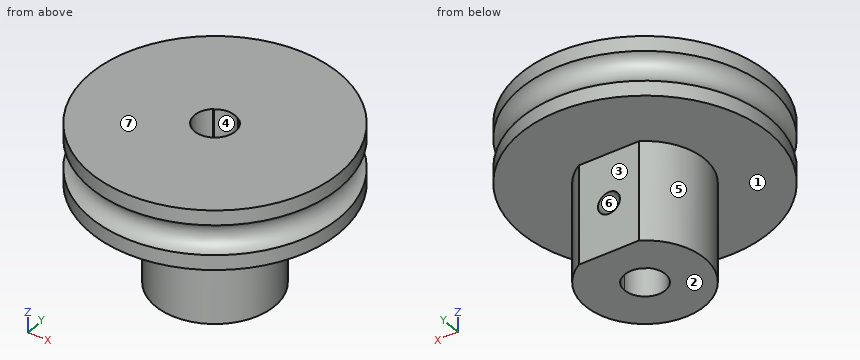
```python
from build123d import *

# Parameters (mm, degrees)
F4_DEPTH = 10
F5_DEPTH = 16.001
F7_D     = 2.2
F7_DEPTH = 4
F8_D     = 4


with BuildPart() as f1:
    # F0 (on Front) → F1 (revolve)
    with BuildSketch(Plane.XZ):
        with BuildLine():
            Line((-12.5, 0), (0, 0))
            Line((0, 0), (0, 6))
            Line((0, 6), (-12.5, 6))
            Line((-12.5, 6), (-12.5, 4.5))
            ThreePointArc((-12.5, 4.5), (-11.3, 3), (-12.5, 1.5))
            Line((-12.5, 1.5), (-12.5, 0))
        make_face()
    revolve(axis=Axis((0, 0, 3), (0, 0, 1)))

    # F3 (on Top) → F4 (join)
    with BuildSketch(Plane.XY):
        with BuildLine():
            Line((3.0351, 5.175729), (-3.0351, 5.175729))
            ThreePointArc((-3.0351, 5.175729), (0, -6), (3.0351, 5.175729))
        make_face()
    extrude(amount=-F4_DEPTH)

    # F2 (on face) → F5 (cut, through all)
    with BuildSketch(Plane.XY.offset(6)):
        with BuildLine():
            ThreePointArc((-1.301243, 1.584066), (-0.876057, -1.853382), (2.05, 0))
            ThreePointArc((2.05, 0), (1.853382, 0.876057), (1.301243, 1.584066))
            Line((1.301243, 1.584066), (-1.301243, 1.584066))
        make_face()
    extrude(amount=-F5_DEPTH, mode=Mode.SUBTRACT)

    # F7
    with Locations(Plane(origin=(0, 5.175729, 0), x_dir=(-1, 0, 0), z_dir=(0, 1, 0))):
        with Locations((0, -5)):
            Hole(F7_D / 2, depth=F7_DEPTH)

    # F8 (through all)
    with Locations(Plane.XY.offset(6)):
        with Locations((0, 0)):
            Hole(F8_D / 2)


solid = f1.part
```
Verification items for the finished model (mm, model axes). Face numbers are marked on the shaded views. A direction names the side the tool comes from. Round coordinates to 2 decimals unless told otherwise and drop trailing zeros. Order: outer loops, then holes, each group sorted by start corner. A loop starts at its lowest first (then second) coordinate and runs counter-clockwise, first axis right, second up. Notation, with made-up numbers: (-15.75, -6) - (38.25, -6) arc R24 ccw to (38.25, 22) - close; hole circle Ø8 at (45.25, -19.75). An arc over 180 degrees is marked (long way). Use CSV: the item, a comma, the result in double quotes.
(1) Gauge pin test, flat ends, axial feed: pin 1 Ø1.5 at (y, z) = (5.5, -2.5) entering from -X; pin 2 Ø2.5 at (x, y) = (0, 0) entering from -Z; pin 3 Ø2 at (x, z) = (5, -8.5) entering from -Y; pin 4 Ø1.3 at (x, z) = (0, -5) entering from -Y. Record the tip position at first contact, or that the pin passes through.
Entries:
pin 1,"x = -3.67"
pin 2,"through"
pin 3,"y = -4.47"
pin 4,"y = -6"
(2) Section check A-A on x = 0. State how many separate pieces and enclosed holes the cut face has, and give its area (3 significant figures).
Entries:
separate pieces,"3"
enclosed holes,"0"
area,"185 mm^2"
(3) Mould release check, pull along Z, two halves, no side actions. Record for the marked faces 5, 6 and 7: released by +Z, released by -Z, zero draft, split by the parting line, or undercut.
Entries:
face 5,"zero draft"
face 6,"undercut"
face 7,"released by +Z"
(4) Access from +Z, -Z, +X, -X, +Y, -Y to the whole of each face (thin tool, end or side, straight path). Record for the marked faces 1, 2, 3 and 4.
Entries:
face 1,"-Z"
face 2,"-Z, +X, -X, +Y, -Y"
face 3,"-Z, +X, -X, +Y"
face 4,"+Z, -Z"
(5) Section check B-B on z = -6.5. Record the boundary of the cut face in (x, y), and give its area (3 significant figures).
Entries:
outline,"(-3.04, 5.18) arc R6 ccw (long way) to (3.04, 5.18) - close; hole (-1.3, 1.58) arc R2.05 ccw (long way) to (2.05, 0) arc R2.05 ccw to (1.3, 1.58) - (1.22, 1.58) arc R2 ccw to (-1.22, 1.58) - close"
area,"96.6 mm^2"
(6) Section check C-C on z = 2.5. Record the boundary of the cut face in (x, y), and give its area (3 significant figures).
Entries:
outline,"circle Ø22.77 at (0, 0); hole (-1.3, 1.58) arc R2.05 ccw (long way) to (2.05, 0) arc R2.05 ccw to (1.3, 1.58) - (1.22, 1.58) arc R2 ccw to (-1.22, 1.58) - close"
area,"394 mm^2"
(7) Thickness scan on probe 1 along Y at (x, z) = (0, -0.5); probe 2 along Z at (x, y) = (0, 3.25); probe 3 along X at (y, z) = (0, -7). Record the ranges inside material, lowest first. Write a range as from..to.
Entries:
probe 1,"-6..-2.05, 2..5.18"
probe 2,"-10..-6.1, -3.9..6"
probe 3,"-6..-2.05, 2.05..6"
